Source: CAD feature listing. Evaluate the final solid. Frame: model axes, mm. Face numbers are marked on the shaded views. A direction names the side the tool comes from. Give positions to 0.01 mm unless a question says otherwise; leave off trailing zeros. Loops run counter-clockwise (first coordinate to the right, second up) from the corner with the lowest first, then second, coordinate; pieces in that order, holes last. Notation, with made-up numbers: (69, 88.25) - (114, 88.25) arc R24 cw to (114, 101.25) - close; hole circle Ø2 at (-35, -27.5). An arc over 180 degrees is marked (long way). Put each result on its own line as item: value.
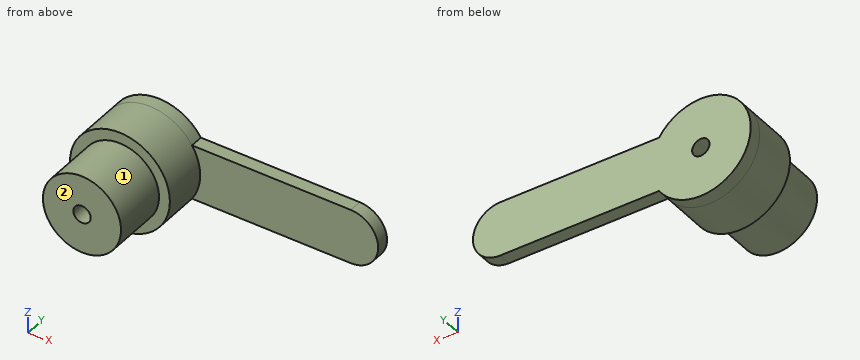
```python
from build123d import *

# Parameters (mm, degrees)
SKETCH1_R           = 2.875
BOSS_EXTRUDE1_DEPTH = 2.55
BOSS_EXTRUDE2_DEPTH = 0.75
SKETCH2_R           = 2.25
BOSS_EXTRUDE3_DEPTH = 3.2
SKETCH3_R           = 0.5
CUT_EXTRUDE1_DEPTH  = 7.5


with BuildPart() as part:
    # Sketch1 → Boss-Extrude1 (new body)
    with BuildSketch(Plane(origin=(0, 0, 0), x_dir=(1, 0, 0), z_dir=(0, 1, 0))):
        Circle(SKETCH1_R)
    extrude(amount=-BOSS_EXTRUDE1_DEPTH)

    # Sketch1<4> → Boss-Extrude2 (add)
    with BuildSketch(Plane(origin=(0, 0, 0), x_dir=(1, 0, 0), z_dir=(0, 1, 0))):
        with BuildLine():
            Line((2.405202694, -1.575), (11.55, -1.575))
            ThreePointArc((11.55, -1.575), (13.125, 0), (11.55, 1.575))
            Line((11.55, 1.575), (2.405202694, 1.575))
            ThreePointArc((2.405202694, 1.575), (-2.875, 0), (2.405202694, -1.575))
        make_face()
    extrude(amount=BOSS_EXTRUDE2_DEPTH)

    # Sketch2 → Boss-Extrude3 (add)
    with BuildSketch(Plane.XZ.offset(2.55)):
        Circle(SKETCH2_R)
    extrude(amount=BOSS_EXTRUDE3_DEPTH)

    # Sketch3 → Cut-Extrude1 (cut, through all)
    with BuildSketch(Plane.XZ.offset(5.75)):
        Circle(SKETCH3_R)
    extrude(amount=-CUT_EXTRUDE1_DEPTH, mode=Mode.SUBTRACT)


solid = part.part
```
1) Material intervals for line 1 along Z through (x, y) = (0, -3.5); line 2 along X through (y, z) = (-2, 0.4); line 3 along Z through (x, y) = (0, -2.25) (3 decimals), sorted ascending. Write a range as [from, to].
Check result:
line 1: [-2.25, -0.5], [0.5, 2.25]
line 2: [-2.85, -0.3], [0.3, 2.85]
line 3: [-2.875, -0.5], [0.5, 2.875]
2) Pin query (flat end, axial travel): P1, Ø2, axis at x = 10, y = -2.5, coming from the -Z side; P2, Ø2.5, axis at x = 9, z = 0.5, coming from the -Y side. Return the tip coordinate at first contact, or that it passes through.
Check result:
P1: through
P2: y = 0
3) Section query B-B, the plane x = 0. Output: boundary loops of the cut face in (y, z) (3 decimals).
Check result:
outline: (-5.75, -2.25) - (-2.55, -2.25) - (-2.55, -2.875) - (0.75, -2.875) - (0.75, -0.5) - (-5.75, -0.5) - close; (-5.75, 0.5) - (0.75, 0.5) - (0.75, 2.875) - (-2.55, 2.875) - (-2.55, 2.25) - (-5.75, 2.25) - close
4) Section query C-C, the plane y = -3.5. Output: boundary loops of the cut face in (x, z).
Check result:
outline: circle Ø4.5 at (0, 0); hole circle Ø1 at (0, 0)
5) Section query D-D, the plane z = -1.8. Output: boundary loops of the cut face in (x, y), plus the area to 3 significant figures.
Check result:
outline: (-2.24, -2.55) - (-1.35, -2.55) - (-1.35, -5.75) - (1.35, -5.75) - (1.35, -2.55) - (2.24, -2.55) - (2.24, 0.75) - (-2.24, 0.75) - close
area: 23.4 mm²
6) Section query A-A, the plane z = 0. Output: boundary loops of the cut face in (x, y) (3 decimals).
Check result:
outline: (-2.875, -2.55) - (-2.25, -2.55) - (-2.25, -5.75) - (-0.5, -5.75) - (-0.5, 0.75) - (-2.875, 0.75) - close; (0.5, -5.75) - (2.25, -5.75) - (2.25, -2.55) - (2.875, -2.55) - (2.875, 0) - (13.125, 0) - (13.125, 0.75) - (0.5, 0.75) - close
7) Access query for the marked faces 1 and 2. Directions: +Z, -Z, +X, -X, +Y, -Y. A direction counts if a zero-diameter tool reaches every point of the face in a straight line with its end or side. Return the directions, or none.
Check result:
face 1: -Y
face 2: +Z, -Z, +X, -X, -Y
